Part model, mm, in its own coordinate system. Face numbers are marked on the shaded views. Give positions to 0.01 mm unless a question says otherwise; leave off trailing zeros. Order: outer loops, then holes, each group sorted by start corner. A loop starts at its lowest first (then second) coordinate and runs counter-clockwise, first axis right, second up. Notation, with made-up numbers: (-4, 31.5) -> (32, 31.5) arc R24 cw to (32, 46.5) -> close; hole circle Ø4 at (80, -38). An arc over 180 degrees is marked (long way). Write item = value, one per line. Start each with the question number.
(1) Saw through at B-B, the plane x = -27. List the corners of the cut face in (y, z).
(2) Flat gauge pins, fed straight in: pin 1 (1.6 mm diameter, centred on x = -23.5, y = -6.5, fed in from +Z); pin 2 (3 mm diameter, centred on x = -28, z = 30.5, fed in from -Y); pin 3 (2.5 mm diameter, centred on x = -19, z = 31, fed in from +Y). Where does each tip first touch, or does it go through?
(3) Probe line 1 along Y through (x, z) = (-25, 37); line 2 along Z through (x, y) = (-20.5, -7.25); line 3 along Z through (x, y) = (-17.75, -11.75). List the from-to ranges inside material, lowest first. Write a range as from..to.
(4) Saw through at C-C, the plane y = -7.25. State how many separate pieces and enclosed holes the cut face has, then the cut area to 3 significant figures.
(5) Two-plate mould, pull along Y, no slides. Class the marked faces 1, 2, 3 and 4: pulls with the +Y half, pulls with the -Y half, needs draft (parallel to the pull), parting line crosses it, or undercut.
Autodesk Inventor part; units mm, degrees
ref_plane "YZ Plane" through (0, 0, 0) normal (1, 0, 0) x (0, 1, 0)
ref_plane "XZ Plane" through (0, 0, 0) normal (0, 1, 0) x (-1, 0, 0)
ref_plane "XY Plane" through (0, 0, 0) normal (0, 0, 1) x (1, 0, 0)
ref_plane "Work Plane1" through (-26.7198, -9.0991, 72.4417) normal (-0.7071068, -0.7071068, 0) x (0.7071068, -0.7071068, 0)
sketch "Sketch1" plane through (-26.7198, -9.0991, 72.4417) normal (-0.7071068, -0.7071068, 0) x (0.7071068, -0.7071068, 0)
  line L0 (-1.6569, 2.5) -> (-1.6569, -60.4376)
  line L1 (-15.5563, 2.5) -> (-1.6569, 2.5)
  line L2 (-15.5563, 2.5) -> (-15.5563, 0)
  line L3 (-7.7782, 0) -> (-15.5563, 0)
  line L4 (-7.7782, -60.4376) -> (-7.7782, 0)
  line L5 (-7.7782, -60.4376) -> (-1.6569, -60.4376)
  circle A0 centre (58.298, -34.4266) radius 35
  line L6 (58.298, -34.4266) -> (-7.7782, -34.4266)
  line L7 (58.298, -34.4266) -> (124.3741, -34.4266) construction
  line L8 (-7.7782, -28.4266) -> (58.298, -28.4266)
  line L9 (58.298, -28.4266) -> (124.3741, -28.4266)
  point P0 (12.4597, -72.4417)
  point P1 (-1.6569, -28.4266)
  point P2 (-7.7782, -28.4266)
  dimension "d0" = 180
  dimension "d1" = 6
extrude "Extrusion1" add sketch "Sketch1" along normal blind 2 contours L0 L6 L4 L8 | L0 L5 L4 L6
sketch "Sketch2" plane through (-27.8914, -7.9275, 12.0041) normal (0, 0, -1) x (-0.7071068, -0.7071068, 0)
  line L0 (0, 6.1213) -> (0, 0)
  line L1 (0, 0) -> (2, 0)
  line L2 (2, 6.1213) -> (2, 0)
  line L3 (0, 6.1213) -> (2, 6.1213)
  point P0 (-25.3278, -14.1166)
extrude "Extrusion2" add sketch "Sketch2" along normal blind 0.2
sketch "Sketch3" plane through (-27.8914, -7.9275, 11.8041) normal (0, 0, -1) x (-0.7071068, 0.7071068, 0)
  arc A0 (-2.8284, 1.1716) -> (0, 0) centre (0, 4) ccw
  line L0 (6.1213, 0) -> (0, 0)
  line L1 (-2.8284, 1.1716) -> (-54.1742, 52.5173)
  line L2 (0, -2) -> (6.1213, -2)
  line L3 (0, 0) -> (0, -2)
  line L4 (-55.5884, 51.1031) -> (-4.2426, -0.2426)
  arc A1 (-4.2426, -0.2426) -> (0, -2) centre (0, 4) ccw
  line L5 (-9.2664, 7.2928) -> (-12.0609, 7.2928)
  line L6 (-9.2664, 7.2928) -> (5.6067, 7.2928)
  line L7 (-12.5609, 16.1266) -> (-12.5609, 10.1266)
  line L8 (-8.9496, 7.2928) -> (-8.9496, 0)
  line L9 (-8.9496, 7.2928) -> (-1.6569, 7.2928) construction
  line L10 (-8.9496, 0) -> (-4.4721, 0)
  line L11 (-8.9496, 0) -> (-4.4721, 0) construction
  point P0 (-14.1166, 25.3278)
  point P1 (-4.4853, 0)
  dimension "d6" = 2
  dimension "d7" = 90
  dimension "d8" = 0
extrude "Extrusion3" add sketch "Sketch3" against normal up to surface (32.211 mm away) contours A0 L3 A1 L4 L8 L1 | L4 L10 L8
sketch "Sketch4" plane through (-27.8914, -7.9275, 11.8041) normal (0, 0, -1) x (-0.7071068, 0.7071068, 0)
  line L0 (6.1213, 0) -> (0, 0)
  arc A0 (-2.8284, 1.1716) -> (0, 0) centre (0, 4) ccw
  line L1 (-2.8284, 1.1716) -> (-8.9496, 7.2928)
  line L2 (-8.9496, 7.2928) -> (-8.9496, 0)
  line L3 (-8.9496, 0) -> (-4.4853, 0)
  line L4 (-4.4853, 0) -> (-4.2426, -0.2426)
  arc A1 (-4.2426, -0.2426) -> (0, -2) centre (0, 4) ccw
  line L5 (0, -2) -> (6.1213, -2)
  line L6 (6.1213, -2) -> (6.1213, 0)
  line L7 (3.1213, 3) -> (6.1213, 0)
  line L8 (-1.1213, 3) -> (3.1213, 3)
  line L9 (-18.8648, 20.7435) -> (-1.1213, 3)
  line L10 (-8.9496, 7.2928) -> (-8.9496, 10.8283)
  point P0 (-14.1166, 25.3278)
extrude "Extrusion4" add sketch "Sketch4" along normal blind 1
fillet "Fillet1" radius 2 1 edges at (-33.634, -5.0133, 27.4096)
sketch "Sketch5" plane through (-21.563, -14.2558, 44.0151) normal (0.7071068, -0.7071068, 0) x (-0.7071068, -0.7071068, 0)
  circle A0 centre (-3.6464, 6) radius 2.5
  point P0 (-25.3278, 44.0151)
extrude "Extrusion5" add sketch "Sketch5" along normal blind 4
chamfer "Chamfer1" distance 0.5 angle 45 1 edges at (-17.2169, -9.9097, 38.0151)
sketch "Sketch6" plane through (-16.1562, -14.5059, 38.0151) normal (0.7071068, -0.7071068, 0) x (-0.7071068, -0.7071068, 0)
  circle A0 centre (0, 0) radius 1.5
  point P0 (-21.6814, 38.0151)
extrude "Extrusion6" cut sketch "Sketch6" against normal through all
sketch "Sketch7" plane through (-28.134, -10.5133, 72.4417) normal (-0.7071068, -0.7071068, 0) x (0, 0, 1)
  line L0 (-61.6376, 5.7782) -> (-28.4266, 5.7782)
  line L1 (-61.6376, 1.6569) -> (-61.6376, 5.7782)
  line L2 (-28.4266, 1.6569) -> (-61.6376, 1.6569)
  line L3 (-28.4266, 1.6569) -> (-28.4266, 5.7782)
  line L4 (-28.4266, 7.7782) -> (-28.4266, 5.7782)
  line L5 (-28.4266, 5.7782) -> (-32.4266, 5.7782)
  line L6 (-32.4266, 5.7782) -> (-32.4266, 1.6569)
  line L7 (-32.4266, 1.6569) -> (-28.4266, 1.6569)
  line L8 (-28.4266, 1.6569) -> (-28.4266, 5.7782)
  circle A0 centre (-34.4873, 3.7175) radius 2.0607
  circle A1 centre (-34.4873, 3.7175) radius 1.5
  point P0 (-72.4417, -12.4597)
  dimension "d21" = 4
  dimension "d22" = 3
extrude "Extrusion7" cut sketch "Sketch7" against normal blind 10 contours A1
sketch "Sketch8" plane through (-28.134, -10.5133, 72.4417) normal (-0.7071068, -0.7071068, 0) x (0, 0, 1)
  circle A0 centre (-34.4873, 3.7175) radius 1.5
  line L0 (-61.6376, 5.7782) -> (-28.4266, 5.7782)
  line L1 (-61.6376, 1.6569) -> (-61.6376, 5.7782)
  line L2 (-28.4266, 1.6569) -> (-61.6376, 1.6569)
  line L3 (-28.4266, 1.6569) -> (-28.4266, 5.7782)
  line L4 (-61.6376, 5.7782) -> (-57.6376, 5.7782)
  line L5 (-57.6376, 5.7782) -> (-57.6376, 1.6569)
  line L6 (-57.6376, 1.6569) -> (-61.6376, 1.6569)
  line L7 (-61.6376, 1.6569) -> (-61.6376, 5.7782)
  circle A1 centre (-55.577, 3.7175) radius 2.0607
  circle A2 centre (-55.577, 3.7175) radius 1.5
  point P0 (-72.4417, -12.4597)
  dimension "d25" = 4
  dimension "d26" = 3
extrude "Extrusion8" cut sketch "Sketch8" against normal blind 10 contours A2
properties part number "GripperHandleRight_3DPrint"
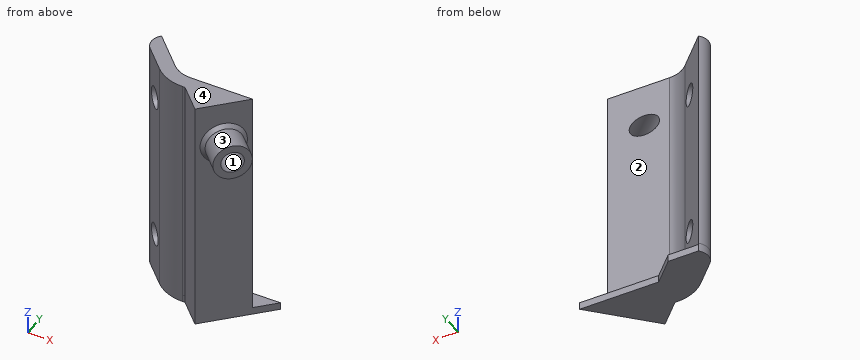
Results list:
q1.outline = (-10.78, 10.8) -> (-4.58, 10.8) -> (-4.58, 11.8) -> (-8.6, 11.8) -> (-8.6, 44.02) -> (-10.78, 44.02) -> close
q2.pin_1 = 11.8
q2.pin_2 = -10.92
q2.pin_3 = -9.1
q3.line_1 = -11.1..-9.1
q3.line_2 = 10.8..11.8
q3.line_3 = 35.65..36.76, 39.27..40.38
q4.separate_pieces = 3
q4.enclosed_holes = 0
q4.area = 92.4 mm^2
q5.face_1 = undercut
q5.face_2 = pulls with the +Y half
q5.face_3 = undercut
q5.face_4 = needs draft
